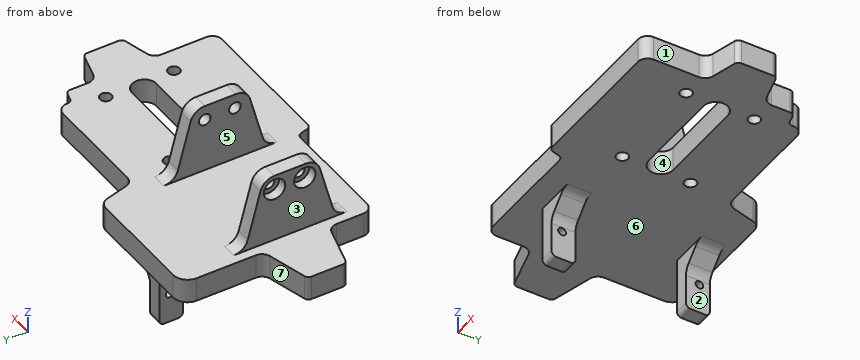
```python
from build123d import *

# Parameters (mm, degrees)
SKETCH1_W                      = 53.5
SKETCH1_H                      = 31.55
BOSS_EXTRUDE1_DEPTH            = 2.5
BOSS_EXTRUDE2_DEPTH            = 5
FILLET1_R                      = 2
FILLET2_R                      = 1
BOSS_EXTRUDE3_DEPTH            = 3
FILLET3_R                      = 3
FILLET3_OF_MIRROR1_R           = 3
SKETCH4_W                      = 3
SKETCH4_H                      = 4.9
BOSS_EXTRUDE4_DEPTH            = 12.3
CHAMFER1_SIZE                  = 4
FILLET4_R                      = 3
FILLET5_R                      = 1
M2_CLEARANCE_HOLE1_D           = 2.4
M2X0_4_TAPPED_HOLE1_D          = 1.6
CBORE_FOR_M2_SHCS1_D           = 2.4
CBORE_FOR_M2_SHCS1_CBORE_D     = 4.4
CBORE_FOR_M2_SHCS1_CBORE_DEPTH = 2
CUT_EXTRUDE1_DEPTH             = 48.058421138


with BuildPart() as part:
    # Sketch1 → Boss-Extrude1 (new, symmetric)
    with BuildSketch(Plane.XY):
        Rectangle(SKETCH1_W, SKETCH1_H)
    extrude(amount=BOSS_EXTRUDE1_DEPTH, both=True)

    # Sketch2 → Boss-Extrude2 (add)
    with BuildSketch(Plane.XY.offset(2.5)):
        with BuildLine():
            Line((-26.75, 20.45), (-26.75, 15.775))
            Line((-26.75, 15.775), (2.056510052, 15.775))
            Line((2.056510052, 15.775), (0, 23.45))
            Line((0, 23.45), (-23.75, 23.45))
            ThreePointArc((-23.75, 23.45), (-25.871320344, 22.571320344), (-26.75, 20.45))
        make_face()
        Polygon((-36.95, 4), (-36.95, -4), (-26.75, -6.733081763), (-26.75, 6.733081763), align=None)
        Polygon((26.75, -15.775), (-2.053847577, -15.775), (-1.25, -18.775), (29.75, -18.775), (29.75, -5.929234186), (36.95, -4), (36.95, 4), (29.75, 5.929234186), (29.75, 12), (26.75, 12.803847577), align=None)
    extrude(amount=-BOSS_EXTRUDE2_DEPTH)

    # Fillet1
    fillet1_edges = [part.edges().sort_by_distance(p)[0] for p in [
        (-26.75, -6.733081763, 0),
        (-26.75, 6.733081763, 0),
        (0, 23.45, 0),
        (2.056510052, 15.775, 0),
        (29.75, -5.929234186, 0),
        (29.75, -18.775, 0),
        (29.75, 5.929234186, 0),
        (-26.75, -15.775, 0),
        (26.75, 15.775, 0),
    ]]
    fillet(fillet1_edges, radius=FILLET1_R)

    # Fillet2
    fillet2_edges = [part.edges().sort_by_distance(p)[0] for p in [
        (-36.95, 4, 0),
        (-36.95, -4, 0),
        (-1.25, -18.775, 0),
        (-2.053847577, -15.775, 0),
        (26.75, 12.803847577, 0),
        (29.75, 12, 0),
        (36.95, 4, 0),
        (36.95, -4, 0),
    ]]
    fillet(fillet2_edges, radius=FILLET2_R)

    # Sketch3 → Boss-Extrude3 (add)
    with BuildSketch(Plane.ZY.offset(21.75)):
        Polygon((16.700757193, -5.5), (16.700757193, 5.5), (2.5, 9.305081422), (2.5, -9.305081422), align=None)
    boss_extrude3 = extrude(amount=BOSS_EXTRUDE3_DEPTH)

    # Fillet3
    fillet3_edges = [part.edges().sort_by_distance(p)[0] for p in [
        (-23.25, -9.305081422, 2.5),
        (-23.25, -5.5, 16.700757193),
        (-23.25, 5.5, 16.700757193),
        (-23.25, 9.305081422, 2.5),
    ]]
    fillet(fillet3_edges, radius=FILLET3_R)

    # Mirror1: Boss-Extrude3 across plane
    add(boss_extrude3.mirror(Plane(origin=(-11.75, 0, 0), x_dir=(0, 0, 1), z_dir=(1, 0, 0))))

    # Fillet3 of Mirror1
    fillet3_of_mirror1_edges = [part.edges().sort_by_distance(p)[0] for p in [
        (-0.25, -9.305081422, 2.5),
        (-0.25, -5.5, 16.700757193),
        (-0.25, 5.5, 16.700757193),
        (-0.25, 9.305081422, 2.5),
    ]]
    fillet(fillet3_of_mirror1_edges, radius=FILLET3_OF_MIRROR1_R)

    # Sketch4 → Boss-Extrude4 (add)
    with BuildSketch(Plane(origin=(0, 0, -2.5), x_dir=(-1, 0, 0), z_dir=(0, 0, -1))):
        with Locations((14.55, 19)):
            Rectangle(SKETCH4_W, SKETCH4_H)
        with Locations((14.55, -8.6)):
            Rectangle(SKETCH4_W, SKETCH4_H)
    extrude(amount=BOSS_EXTRUDE4_DEPTH)

    # Chamfer1
    chamfer1_edges = [part.edges().sort_by_distance(p)[0] for p in [
        (-13.05, 19, -2.5),
        (-13.05, -8.6, -2.5),
    ]]
    chamfer(chamfer1_edges, length=CHAMFER1_SIZE)

    # Fillet4
    fillet4_edges = [part.edges().sort_by_distance(p)[0] for p in [
        (-13.05, -8.6, -6.5),
        (-9.05, 19, -2.5),
        (-9.05, -8.6, -2.5),
        (-13.05, 19, -6.5),
    ]]
    fillet(fillet4_edges, radius=FILLET4_R)

    # Fillet5
    fillet5_edges = [part.edges().sort_by_distance(p)[0] for p in [
        (-14.55, 16.55, -14.8),
        (-14.55, 21.45, -14.8),
        (-14.55, -11.05, -14.8),
        (-14.55, -6.15, -14.8),
    ]]
    fillet(fillet5_edges, radius=FILLET5_R)

    # M2 Clearance Hole1 (through all)
    with Locations(Plane.XY.offset(2.5)):
        with Locations((3.75, 7), (3.75, -7), (24.75, -7), (24.75, 7)):
            Hole(M2_CLEARANCE_HOLE1_D / 2)

    # M2x0.4 Tapped Hole1 (through all)
    with Locations(Plane.ZY.offset(16.05)):
        with Locations((-8.65, 19.3), (-8.65, -8.9)):
            Hole(M2X0_4_TAPPED_HOLE1_D / 2)

    # CBORE for M2 SHCS1 (through all)
    with Locations(Plane.ZY.offset(24.75)):
        with Locations((13.700757193, 3.198019036), (13.700757193, -3)):
            CounterBoreHole(CBORE_FOR_M2_SHCS1_D / 2, CBORE_FOR_M2_SHCS1_CBORE_D / 2, CBORE_FOR_M2_SHCS1_CBORE_DEPTH)

    # Sketch13 → Cut-Extrude1 (cut, through all)
    with BuildSketch(Plane.XY.offset(2.5)):
        with BuildLine():
            Line((5.25, 2.5), (23.25, 2.5))
            ThreePointArc((23.25, 2.5), (25.75, 0), (23.25, -2.5))
            Line((23.25, -2.5), (5.25, -2.5))
            ThreePointArc((5.25, -2.5), (2.75, 0), (5.25, 2.5))
        make_face()
    extrude(amount=-CUT_EXTRUDE1_DEPTH, mode=Mode.SUBTRACT)


solid = part.part
```
Check sheet for the modelled part. Datum: model origin and axes. Units: mm. Face numbers are marked on the shaded views. A direction names the side the tool comes from. Give positions to 0.01 mm unless a question says otherwise; leave off trailing zeros. Loops run counter-clockwise (first coordinate to the right, second up) from the corner with the lowest first, then second, coordinate; pieces in that order, holes last. Notation, with made-up numbers: M -23.5,-22.75 L -0.5,-22.75 A21 cw -0.5,-14.75 Z; hole C 27,17 d7. An arc over 180 degrees is marked long. Answer as CSV lines item,"result".
Item 1: Set-up check for the marked faces 1, 2 and 3: record each of +Z, -Z, +X, -X, +Y, -Y from which the full face is reachable in a straight line by a thin tool's end or side.
Reply:
face 1,"+Z, -Z, +X, -Y"
face 2,"-Z, +X, +Y, -Y"
face 3,"+Z, -X, +Y, -Y"
Item 2: Sectioned sample at C-C, the plane z = 0. State how many separate pieces and enclosed holes the cut face has, then the cut area to 3 significant figures.
Reply:
separate pieces,"1"
enclosed holes,"5"
area,"2,130 mm^2"
Item 3: Sectioned sample at B-B, the plane z = -8.65. Enter the section's corners in (x, y).
Reply:
outline,"M -16.05,-11.05 L -13.05,-11.05 L -13.05,-9.7 L -16.05,-9.7 Z; M -16.05,-8.1 L -13.05,-8.1 L -13.05,-6.15 L -16.05,-6.15 Z; M -16.05,16.55 L -13.05,16.55 L -13.05,18.5 L -16.05,18.5 Z; M -16.05,20.1 L -13.05,20.1 L -13.05,21.45 L -16.05,21.45 Z"
Item 4: Sectioned sample at A-A, the plane x = 17. Enter the section's corners in (y, z) (3 decimals).
Reply:
outline,"M -18.775,-2.5 L -2.5,-2.5 L -2.5,2.5 L -18.775,2.5 Z; M 2.5,-2.5 L 15.775,-2.5 L 15.775,2.5 L 2.5,2.5 Z"
Item 5: Sectioned sample at D-D, the plane y = 10. Enter the section's corners in (x, z).
Reply:
outline,"M -26.75,-2.5 L 29.75,-2.5 L 29.75,2.5 L 1.25,2.5 L 1.25,2.97 L -1.75,2.97 L -1.75,2.5 L -21.75,2.5 L -21.75,2.97 L -24.75,2.97 L -24.75,2.5 L -26.75,2.5 Z"
Item 6: Scan lines: L1, parallel to Y at x = -15.05, z = -8.65; L2, parallel to X at y = -1, z = 12; L3, parallel to Z at x = -29, y = -0.5. Record each from-to range of solid material in increasing order.
Reply:
L1,"-11.05 to -9.7, -8.1 to -6.15, 16.55 to 18.5, 20.1 to 21.45"
L2,"-24.75 to -21.75, -1.75 to 1.25"
L3,"-2.5 to 2.5"
Item 7: Draft check along X on the marked faces 4, 5, 6 and 7. Enter one of: pulls with the +X half, pulls with the -X half, needs draft (parallel to the pull), parting line crosses it, or undercut.
Reply:
face 4,"undercut"
face 5,"undercut"
face 6,"needs draft"
face 7,"pulls with the -X half"
Item 8: Depth check by flat-ended pin: pin 1 Ø8 at (x, y) = (-13.5, 12) entering from -Z; pin 2 Ø3 at (y, z) = (-3, 13.7) entering from -X; pin 3 Ø2.5 at (y, z) = (18.5, -9.5) entering from +X; pin 4 Ø2 at (x, y) = (24.75, -7) entering from +Z. Enter the tip coordinate at first touch or a pass-through.
Reply:
pin 1,"z = -2.5"
pin 2,"x = -22.75"
pin 3,"x = -13.05"
pin 4,"through"
